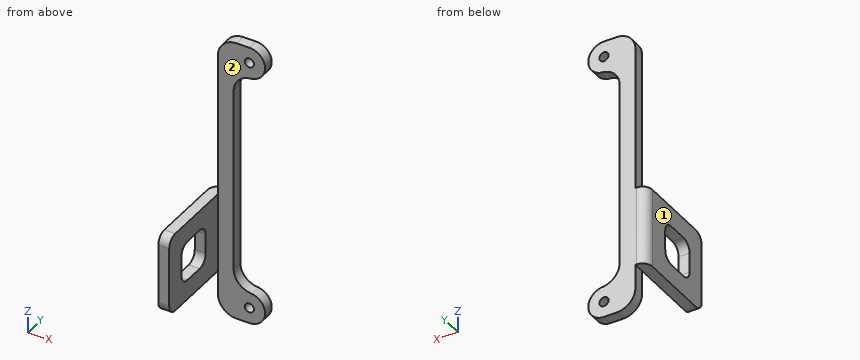
Autodesk Inventor part; units mm, degrees
ref_plane "YZ Plane" through (0, 0, 0) normal (1, 0, 0) x (0, 1, 0)
ref_plane "XZ Plane" through (0, 0, 0) normal (0, 1, 0) x (-1, 0, 0)
ref_plane "XY Plane" through (0, 0, 0) normal (0, 0, 1) x (1, 0, 0)
sketch "Sketch1" plane through (0, 0, 0) normal (0, 1, 0) x (-1, 0, 0)
  circle A0 centre (0, 0) radius 1.4732
  circle A1 centre (0, -80.9498) radius 1.4732
  circle A2 centre (0, 0) radius 5.0165
  circle A3 centre (0, -80.9498) radius 5.0165
  line L0 (0, 5.0165) -> (4.033, 5.0165)
  line L1 (4.033, -85.9663) -> (0, -85.9663)
  line L2 (10.033, -79.9663) -> (10.033, -0.9835)
  line L3 (0, -5.0165) -> (-0.9835, -5.0165)
  line L4 (5.0165, -11.0165) -> (5.0165, -69.9333)
  line L5 (-0.9835, -75.9333) -> (0, -75.9333)
  arc A4 (10.033, -0.9835) -> (4.033, 5.0165) centre (4.033, -0.9835) ccw
  arc A5 (4.033, -85.9663) -> (10.033, -79.9663) centre (4.033, -79.9663) ccw
  arc A6 (5.0165, -11.0165) -> (-0.9835, -5.0165) centre (-0.9835, -11.0165) ccw
  arc A7 (-0.9835, -75.9333) -> (5.0165, -69.9333) centre (-0.9835, -69.9333) ccw
  point P0 (10.033, 5.0165)
  dimension "d0" = 2.9464
  dimension "d2" = 2.9464
  dimension "d3" = 10.033
  dimension "d4" = 10.033
  dimension "d7" = 80.9498
  dimension "d8" = 10.033
  dimension "d9" = 6
  dimension "d10" = 6
  dimension "d11" = 6
  dimension "d12" = 6
extrude "Extrusion1" add sketch "Sketch1" along normal blind 3.5
sketch "Sketch2" plane through (-10.033, 0, -79.9663) normal (-1, 0, 0) x (0, 0, 1)
  line L0 (0, 0) -> (0, 3.5)
  line L1 (0, 0) -> (7.62, 0)
  line L2 (0, 0) -> (78.9828, 0)
  line L3 (7.62, 0) -> (7.62, -22.225)
  line L4 (7.62, 0) -> (33.02, 0)
  line L5 (68.9498, 0) -> (10.033, 0)
  line L6 (33.02, 0) -> (33.02, -22.225)
  line L7 (29.845, -25.4) -> (10.795, -25.4)
  line L8 (7.62, 0) -> (19.2419, 0) construction
  line L9 (33.02, 0) -> (44.6419, 0) construction
  line L10 (23.495, -6.35) -> (17.145, -6.35)
  line L11 (17.145, -19.05) -> (23.495, -19.05)
  line L12 (26.67, -15.875) -> (26.67, -9.525)
  line L13 (13.97, -9.525) -> (13.97, -15.875)
  arc A0 (17.145, -6.35) -> (13.97, -9.525) centre (17.145, -9.525) ccw
  arc A1 (26.67, -9.525) -> (23.495, -6.35) centre (23.495, -9.525) ccw
  arc A2 (23.495, -19.05) -> (26.67, -15.875) centre (23.495, -15.875) ccw
  arc A3 (13.97, -15.875) -> (17.145, -19.05) centre (17.145, -15.875) ccw
  arc A4 (7.62, -22.225) -> (10.795, -25.4) centre (10.795, -22.225) ccw
  arc A5 (29.845, -25.4) -> (33.02, -22.225) centre (29.845, -22.225) ccw
  line L14 (78.9828, 0) -> (78.9828, 3.5)
  point P0 (79.9663, 0)
  point P1 (7.62, -25.4)
  point P2 (13.97, -6.35)
  point P3 (33.02, 0)
  point P4 (78.9828, 1.75)
  dimension "d15" = 7.62
  dimension "d16" = 25.4
  dimension "d17" = 25.4
  dimension "d19" = 6.35
  dimension "d22" = 3.175
  dimension "d23" = 3.175
  dimension "d24" = 3.175
  dimension "d25" = 3.175
  dimension "d26" = 3.175
  dimension "d27" = 3.175
  dimension "d33" = 78.9828
extrude "Extrusion2" add sketch "Sketch2" along normal blind 3.5
sketch "Sketch4" plane through (-10.033, 0, -46.9463) normal (0, 1, 0) x (1, 0, 0)
  line L0 (0, 25.4) -> (-3.5, 25.4)
  line L1 (0, 25.4) -> (-3.5, 25.4)
  line L2 (0, 0) -> (-3.5, 0)
  line L3 (-3.5, 25.4) -> (-3.5, 0)
  line L4 (-3.5, 0) -> (0, 0)
  line L5 (0, 0) -> (0, 25.4)
  point P0 (10.033, -46.9463)
extrude "Extrusion3" add sketch "Sketch4" along normal blind 3.5
fillet "Fillet1" radius 3.175 1 edges at (-13.533, 3.5, -59.6463)
properties part number "sidemount1_3DPrint"
Read the model definition and answer for the solid it produces. Units are mm, in the model's axes. Face numbers are marked on the shaded views. A direction names the side the tool comes from. Give positions to 0.01 mm unless a question says otherwise; leave off trailing zeros. Write each loop counter-clockwise with the first axis right and the second up, starting at its lowest first coordinate (ties: lowest second). Pieces come first, ordered by that corner, then holes. Notation, with made-up numbers: (12, -32) - (57, -32) arc R11 ccw to (57, -22) - close; hole circle Ø4 at (88, 85). An arc over 180 degrees is marked (long way). Use CSV: the item, a comma, the result in double quotes. Start each with the question number.
(1) For the marked faces 1 and 2, determine the directions among +Z, -Z, +X, -X, +Y, -Y from which every point of the face is accessible in a straight line to the end or side of a thin tool.
(2) Find section C-C (z = -31.5). Give the vertices of the cut face in (x, y).
(3) Find section A-A (y = -13). Give the vertices of the cut face in (x, z), plus the area to 4 significant figures.
(4) Consider line 1 along X through (y, z) = (2.5, -80); line 2 along X through (y, z) = (-0.75, -66.5); line 3 along X through (y, z) = (2, -23). Determine where each line is inside the solid, lowest interval first.
(5) Given P1, Ø4, axis at x = -12.5, y = -11.5, coming from the +Z side; P2, Ø4, axis at x = -12.5, y = -14, coming from the -Z side; P3, Ø4, axis at y = 2, z = -13, coming from the -X side; P4, Ø1.5, axis at y = -2.5, z = -26, coming from the +X side (1 decimal), each flat-ended and moving along its own axis, determine where each tip first touches the part or whether it passes through.
(6) Find section D-D (y = -20.5). Give the vertices of the cut face in (x, z), plus the area to 3 significant figures.
(7) Find section B-B (z = 0). Give the vertices of the cut face in (x, y).
Findings below:
1,face 1,"+Z, -Z, -X, +Y, -Y"
1,face 2,"+Z, -Z, +X, -Y"
2,outline,"(-10.03, 0) - (-5.02, 0) - (-5.02, 3.5) - (-10.03, 3.5) - close"
3,outline,"(-13.53, -72.35) - (-10.03, -72.35) - (-10.03, -66) - (-13.53, -66) - close; (-13.53, -53.3) - (-10.03, -53.3) - (-10.03, -46.95) - (-13.53, -46.95) - close"
3,area,"44.45 mm2"
4,line 1,"-10.03 to -1.13, 1.13 to 4.93"
4,line 2,"-13.53 to -10.03"
4,line 3,"-10.03 to -5.02"
5,P1,"z = -46.95"
5,P2,"z = -72.35"
5,P3,"x = -10.03"
5,P4,"through"
6,outline,"(-13.53, -72.35) - (-10.03, -72.35) - (-10.03, -46.95) - (-13.53, -46.95) - close"
6,area,"88.9 mm2"
7,outline,"(-9.95, 0) - (-1.47, 0) - (-1.47, 3.5) - (-9.95, 3.5) - close; (1.47, 0) - (5.02, 0) - (5.02, 3.5) - (1.47, 3.5) - close"
